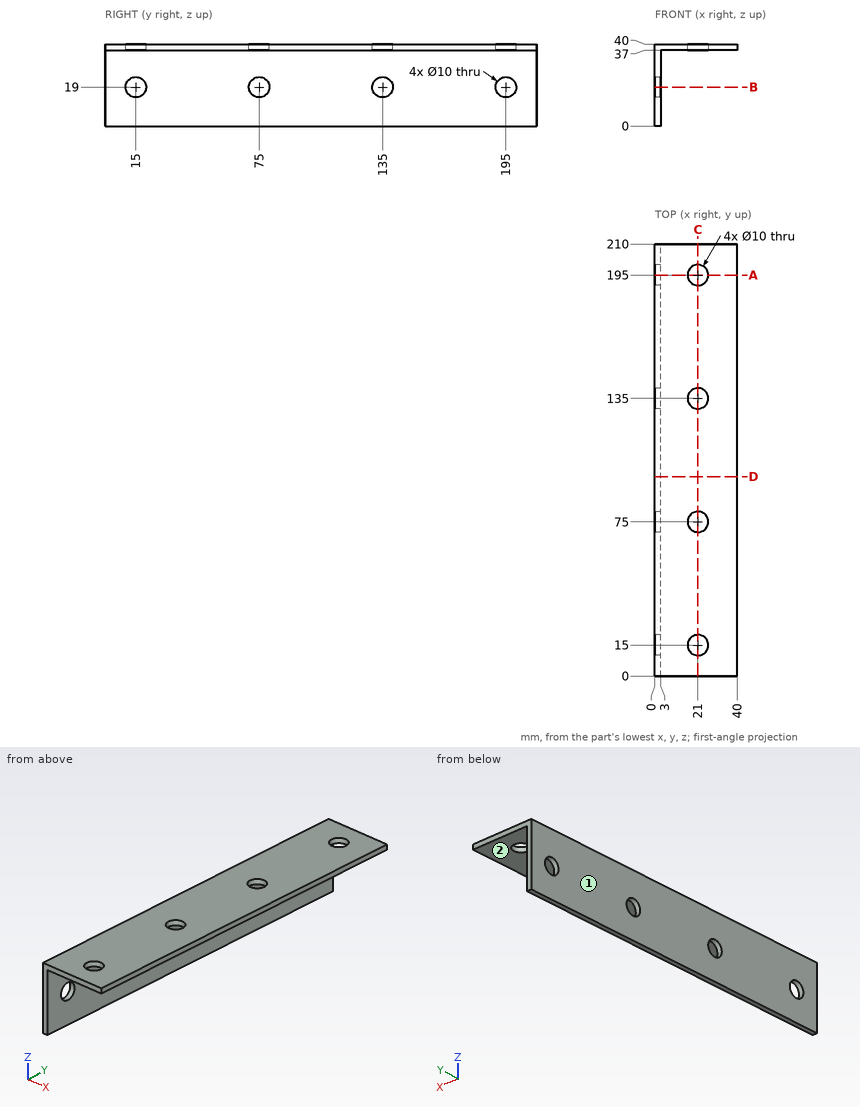
Geometry check sheet. Reference: drawing and pictorial views, mm from the part's lowest x, y, z. A direction names the side the tool comes from. Coordinates: 2 decimals unless noted, no trailing zeros. Order: outer loops, then holes, each group sorted by start corner. A loop starts at its lowest first (then second) coordinate and runs counter-clockwise, first axis right, second up. Notation, with made-up numbers: (1, 44) -> (9, 44) arc R15 ccw to (9, 58) -> close; hole circle Ø4 at (-31, 41.25). An arc over 180 degrees is marked (long way). Write item = value, one per line. Start each with the question number.
1) Cross-section at D-D (y = 97). Enter the section's corners in (x, z), then the cut area to 3 significant figures.
2) Cross-section at A-A (y = 195). Enter the section's corners in (x, z), then the cut area to 3 significant figures.
3) Cross-section at B-B (z = 19). Enter the section's corners in (x, y), then the cut area to 3 significant figures.
4) Cross-section at C-C (x = 21). Enter the section's corners in (y, z), then the cut area to 3 significant figures.
5) Access from +Z, -Z, +X, -X, +Y, -Y to the whole of each face (thin tool, end or side, straight path). Record for the marked faces 1 and 2.
6) Go/stop test with flat-tipped pins: P1, Ø6, axis at y = 99.5, z = 19.5, coming from the +X side; P2, Ø6, axis at y = 135, z = 19, coming from the -X side; P3, Ø5, axis at y = 187, z = 19, coming from the -X side; P4, Ø5, axis at x = 10.5, y = 168.5, coming from the -Z side. Record where each tip stops, or that it passes through.
7) Material ranges on L1, parallel to Y at x = 0.85, z = 19; L2, parallel to Z at x = 28, y = 181; L3, parallel to X at y = 32.5, z = 18.5, recorded low to high.
Ans:
q1.outline = (0, 0) -> (3, 0) -> (3, 37) -> (40, 37) -> (40, 40) -> (0, 40) -> close
q1.area = 231 mm²
q2.outline = (0, 0) -> (3, 0) -> (3, 14) -> (0, 14) -> close; (0, 24) -> (3, 24) -> (3, 37) -> (16, 37) -> (16, 40) -> (0, 40) -> close; (26, 37) -> (40, 37) -> (40, 40) -> (26, 40) -> close
q2.area = 171 mm²
q3.outline = (0, 0) -> (3, 0) -> (3, 10) -> (0, 10) -> close; (0, 20) -> (3, 20) -> (3, 70) -> (0, 70) -> close; (0, 80) -> (3, 80) -> (3, 130) -> (0, 130) -> close; (0, 140) -> (3, 140) -> (3, 190) -> (0, 190) -> close; (0, 200) -> (3, 200) -> (3, 210) -> (0, 210) -> close
q3.area = 510 mm²
q4.outline = (0, 37) -> (10, 37) -> (10, 40) -> (0, 40) -> close; (20, 37) -> (70, 37) -> (70, 40) -> (20, 40) -> close; (80, 37) -> (130, 37) -> (130, 40) -> (80, 40) -> close; (140, 37) -> (190, 37) -> (190, 40) -> (140, 40) -> close; (200, 37) -> (210, 37) -> (210, 40) -> (200, 40) -> close
q4.area = 510 mm²
q5.face_1 = +Z, -Z, -X, +Y, -Y
q5.face_2 = -Z, +X, +Y, -Y
q6.P1 = 3
q6.P2 = through
q6.P3 = 0
q6.P4 = 37
q7.L1 = 0 to 10, 20 to 70, 80 to 130, 140 to 190, 200 to 210
q7.L2 = 37 to 40
q7.L3 = 0 to 3
